Input: part model. Units: mm. Frame: model coordinates. A direction names the side the tool comes from. Give positions to 0.01 mm unless a question says otherwise; leave off trailing zeros. Loops run counter-clockwise (first coordinate to the right, second up) from the corner with the lowest first, then second, coordinate; pieces in that order, holes last. Notation, with made-up numbers: M 31,9 L 65,9 A21 cw 65,16 Z; hole C 11.5,53.25 d10. An arc over 180 degrees is marked long. Use a Markdown table: item, result. Add a question column.
from build123d import *

# Parameters (mm, degrees)
SKETCH1_R           = 5.25
SKETCH1_R_2         = 1.5
BOSS_EXTRUDE4_DEPTH = 13
FILLET2_R           = 4
FILLET3_R           = 4
SKETCH2_R           = 1.65
CUT_EXTRUDE1_DEPTH  = 40.402671632


with BuildPart() as part:
    # Sketch1 → Boss-Extrude4 (new body)
    with BuildSketch(Plane(origin=(0, 0, 0), x_dir=(1, 0, 0), z_dir=(0, 1, 0))):
        with BuildLine():
            Line((-16.582575695, 10), (-29.23303836, 10))
            Line((-29.23303836, 10), (-29.23303836, -12))
            Line((-29.23303836, -12), (25.76696164, -12))
            Line((25.76696164, -12), (25.76696164, -1))
            Line((25.76696164, -1), (19.533923281, -1))
            ThreePointArc((19.533923281, -1), (11.498909656, -7.583462828), (4.4, 0))
            Line((4.4, 0), (-1, 0))
            ThreePointArc((-1, 0), (-6.058970318, 9.257654472), (-16.582575695, 10))
        make_face()
        with Locations(Location((-12, 0, 0), (0, 0, 90))):
            Circle(SKETCH1_R, mode=Mode.SUBTRACT)
        with Locations(Location((-4, 0, 0), (0, 0, 90))):
            Circle(SKETCH1_R_2, mode=Mode.SUBTRACT)
        with Locations(Location((-20, 0, 0), (0, 0, 90))):
            Circle(SKETCH1_R_2, mode=Mode.SUBTRACT)
    extrude(amount=BOSS_EXTRUDE4_DEPTH)

    # Fillet2
    fillet2_edges = [part.edges().sort_by_distance(p)[0] for p in [
        (25.76696164, 13, 6.5),
    ]]
    fillet(fillet2_edges, radius=FILLET2_R)

    # Fillet3
    fillet3_edges = [part.edges().sort_by_distance(p)[0] for p in [
        (-29.23303836, 6.5, -10),
    ]]
    fillet(fillet3_edges, radius=FILLET3_R)

    # Sketch2 → Cut-Extrude1 (cut, through all)
    with BuildSketch(Plane.XY.offset(12)):
        with Locations((22.26696164, 6.5)):
            Circle(SKETCH2_R)
        with Locations((1.73303836, 6.5)):
            Circle(SKETCH2_R)
        with Locations((-22.73, 6.761910465)):
            Circle(SKETCH2_R)
    extrude(amount=-CUT_EXTRUDE1_DEPTH, mode=Mode.SUBTRACT)


solid = part.part
1) Ray query, line 1 (Z direction, x = -20, y = 10.25); line 2 (Y direction, x = -22.73, z = 1); line 3 (X direction, y = 11.25, z = 0.5). Return the intervals inside material, ascending. Write a range as [from, to].
2) Reachability of faces 1 (the flat face through (-21, 6, -10)), 2 (the flat face through (4, 6, 0)), 3 (the cylindrical face through (-4.45, 6.41, -1.43)) from +Z, -Z, +X, -X, +Y, -Y: full face, straight path, thin tool, end or side. Return the list, or none.
3) Section query D-D, the plane y = 9.5. Return the cut outline in (x, z), and give its area (3 significant figures).
4) Section query A-A, the plane x = -12. Return the cut outline in (y, z).
5) Contact query for flat-ended pins moving along their axis: P1, Ø2, axis at y = 9.5, z = -6.5, coming from the +X side; P2, Ø7, axis at x = -23, y = 7.5, coming from the -Z side; P3, Ø4, axis at x = 0, y = 5.5, coming from the -Z side; P4, Ø2, axis at x = 1.73, y = 6.5, coming from the -Z side. Output: stop coordinate, or through.
6) Section query B-B, the plane y = 1. Return the cut outline in (x, z).
7) Pull-direction query (Y, two-part tool) for faces 4 (the cylindrical face through (24.626, 11.797, 6.423)), 5 (the flat face through (23.4, 5, 1)), 6 (the flat face through (-8, 0, 5)), 7 (the cylindrical face through (23.79, 5.87, 6.58)); classes: pulls with the +Y half, pulls with the -Y half, needs draft (parallel to the pull), parting line crosses it, or undercut.
8) Section query C-C, the plane x = -22.73. Return the cut outline in (y, z), and give its area (3 significant figures).
Entries:
| question | item | result |
|---|---|---|
| 1 | line 1 | z = [-10, -1.5], [1.5, 12] |
| 1 | line 2 | y = [0, 5.11], [8.41, 13] |
| 1 | line 3 | x = [-29.23, -21.41], [-18.59, -17.23], [-6.77, -5.41], [-2.59, 4.42] |
| 2 | face 1 | -Z, -X, +Y, -Y |
| 2 | face 2 | -Z, +X, +Y, -Y |
| 2 | face 3 | +Y, -Y |
| 3 | outline | M -29.23,-6 A4 ccw -25.23,-10 L -16.58,-10 A11 ccw -1,0 L 4.4,0 A7.6 cw 19.53,1 L 25.74,1 L 25.74,12 L -29.23,12 Z; hole C -20,0 d3; hole C -12,0 d10.5; hole C -4,0 d3 |
| 3 | area | 729 mm² |
| 4 | outline | M 0,-11 L 13,-11 L 13,-5.25 L 0,-5.25 Z; M 0,5.25 L 13,5.25 L 13,12 L 0,12 Z |
| 5 | P1 | stops at x = -2.47 |
| 5 | P2 | stops at z = -10 |
| 5 | P3 | stops at z = -4.58 |
| 5 | P4 | passes through |
| 6 | outline | M -29.23,-6 A4 ccw -25.23,-10 L -16.58,-10 A11 ccw -1,0 L 4.4,0 A7.6 cw 19.53,1 L 25.77,1 L 25.77,12 L -29.23,12 Z; hole C -20,0 d3; hole C -12,0 d10.5; hole C -4,0 d3 |
| 7 | face 4 | pulls with the +Y half |
| 7 | face 5 | needs draft |
| 7 | face 6 | pulls with the -Y half |
| 7 | face 7 | undercut |
| 8 | outline | M 0,-10 L 5.11,-10 L 5.11,12 L 0,12 Z; M 8.41,-10 L 13,-10 L 13,12 L 8.41,12 Z |
| 8 | area | 213 mm² |
